Part model, mm, in its own coordinate system. A direction names the side the tool comes from. Round coordinates to 2 decimals unless told otherwise and drop trailing zeros. Write each loop counter-clockwise with the first axis right and the second up, starting at its lowest first coordinate (ties: lowest second). Pieces come first, ordered by that corner, then holes. Notation, with made-up numbers: M -34.75,3.5 L -5.75,3.5 A14 cw -5.75,17.5 Z; hole C -1.5,65.5 d1. An arc over 180 degrees is marked long. One line per question, with ' | ' between items. Start each with the question number.
1) Drop flat-ended pins along their axis: pin 1 Ø2.5 at (x, z) = (-22.5, 2) entering from +Y; pin 2 Ø2.5 at (x, z) = (-23, 1.5) entering from -Y; pin 3 Ø3 at (x, z) = (5, 2) entering from +Y. Give the stop position or say it passes through.
2) Saw through at C-C (y = -35). List the corners of the cut face in (x, z) (3 decimals), plus the area to 3 significant figures.
3) Saw through at B-B (x = -19). List the corners of the cut face in (y, z) (3 decimals), plus the area to 3 significant figures.
4) Mould opens along Y. For faces 1 (the face through (-29, -1.325, 2)), 2 (the face through (4, 0, 0)), 3 (the face through (-59.94, 2.64, 2.46)) say: pulls with the +Y half, pulls with the -Y half, needs draft (parallel to the pull), parting line crosses it, or undercut.
5) Wall check: probe 1 along X at (y, z) = (-24.5, 2.65) (3 decimals); probe 2 along Y at (x, z) = (24, 2.85) (3 decimals); probe 3 along Y at (x, z) = (18.5, 2.3) (3 decimals). Give the ranges that are in metal, low to high. Write a range as [from, to].
6) Tool access for faces 4 (the face through (-28, 1.325, 2)), 5 (the face through (4, 0, 5)): list every direction of +Z, -Z, +X, -X, +Y, -Y with a clear straight run to the whole face (end or side of a thin tool).
7) Saw through at A-A (z = 2.1). List the corners of the cut face in (x, y) (3 decimals), plus the area to 3 significant figures.
```python
from build123d import *

# Parameters (mm, degrees)
SKETCH1_R           = 60
SKETCH1_R_2         = 3
BOSS_EXTRUDE2_DEPTH = 5


with BuildPart() as part:
    # Sketch1 → Boss-Extrude2 (new body)
    # profile 1 of 2: a face of its own
    with BuildSketch(Plane.XY):
        Circle(SKETCH1_R)
        with BuildLine():
            Line((-1.325, 54.984037456), (-1.325, 2.691537665))
            ThreePointArc((-1.325, 2.691537665), (0, 3), (1.325, 2.691537665))
            Line((1.325, 2.691537665), (1.325, 54.984037456))
            ThreePointArc((1.325, 54.984037456), (38.890872965, 38.890872965), (54.984037456, 1.325))
            Line((54.984037456, 1.325), (2.691537665, 1.325))
            ThreePointArc((2.691537665, 1.325), (2.921866954, 0.680215777), (3, 0))
            ThreePointArc((3, 0), (2.921866954, -0.680215777), (2.691537665, -1.325))
            Line((2.691537665, -1.325), (54.984037456, -1.325))
            ThreePointArc((54.984037456, -1.325), (38.890872965, -38.890872965), (1.325, -54.984037456))
            Line((1.325, -54.984037456), (1.325, -2.691537665))
            ThreePointArc((1.325, -2.691537665), (0, -3), (-1.325, -2.691537665))
            Line((-1.325, -2.691537665), (-1.325, -54.984037456))
            ThreePointArc((-1.325, -54.984037456), (-38.890872965, -38.890872965), (-54.984037456, -1.325))
            Line((-54.984037456, -1.325), (-2.691537665, -1.325))
            ThreePointArc((-2.691537665, -1.325), (-3, 0), (-2.691537665, 1.325))
            Line((-2.691537665, 1.325), (-54.984037456, 1.325))
            ThreePointArc((-54.984037456, 1.325), (-38.890872965, 38.890872965), (-1.325, 54.984037456))
        make_face(mode=Mode.SUBTRACT)
    # profile 2 of 2: a face of its own
    with BuildSketch(Plane.XY):
        Circle(SKETCH1_R_2)
        with BuildLine():
            ThreePointArc((-1.325, 1.498123827), (0, -2), (1.325, 1.498123827))
            Line((1.325, 1.498123827), (-1.325, 1.498123827))
        make_face(mode=Mode.SUBTRACT)
    extrude(amount=BOSS_EXTRUDE2_DEPTH)


solid = part.part
```
Answer key:
1) pin 1: stops at y = 56.11 | pin 2: stops at y = -55.92 | pin 3: stops at y = 59.9
2) outline: M -48.734,0 L -42.426,0 L -42.426,5 L -48.734,5 Z; M -1.325,0 L 1.325,0 L 1.325,5 L -1.325,5 Z; M 42.426,0 L 48.734,0 L 48.734,5 L 42.426,5 Z | area: 76.3 mm2
3) outline: M -56.912,0 L -51.614,0 L -51.614,5 L -56.912,5 Z; M -1.325,0 L 1.325,0 L 1.325,5 L -1.325,5 Z; M 51.614,0 L 56.912,0 L 56.912,5 L 51.614,5 Z | area: 66.2 mm2
4) face 1: undercut | face 2: needs draft | face 3: parting line crosses it
5) probe 1: x = [-54.77, -49.242], [-1.325, 1.325], [49.242, 54.77] | probe 2: y = [-54.991, -49.487], [-1.325, 1.325], [49.487, 54.991] | probe 3: y = [-57.077, -51.795], [-1.325, 1.325], [51.795, 57.077]
6) face 4: +Z, -Z | face 5: +Z, +X, -X, +Y, -Y
7) outline: C 0,0 d120; hole M -54.984,-1.325 A55 ccw -1.325,-54.984 L -1.325,-2.692 A3 cw -2.692,-1.325 Z; hole M -54.984,1.325 L -2.692,1.325 A3 cw -1.325,2.692 L -1.325,54.984 A55 ccw Z; hole M -1.325,1.498 A2 ccw long 1.325,1.498 Z; hole M 1.325,-54.984 A55 ccw 54.984,-1.325 L 2.692,-1.325 A3 cw 1.325,-2.692 Z; hole M 1.325,2.692 A3 cw 2.692,1.325 L 54.984,1.325 A55 ccw 1.325,54.984 Z | area: 2,380 mm2
